from build123d import *

# Parameters (mm, degrees)
F0_R     = 48.25
F0_R_2   = 46.25
F0_R_3   = 43
F0_R_4   = 41
F1_DEPTH = 5
F2_DEPTH = 4.75
F3_SIZE  = 0.3


with BuildPart() as f1:
    # F0 (on Front) → F1 (new body, symmetric)
    with BuildSketch(Plane.XZ):
        Circle(F0_R)
        Circle(F0_R_2, mode=Mode.SUBTRACT)
        Circle(F0_R_3)
        Circle(F0_R_4, mode=Mode.SUBTRACT)
    extrude(amount=F1_DEPTH, both=True)

    # F0 (on Front) → F2 (join, symmetric)
    with BuildSketch(Plane.XZ):
        Circle(F0_R_2)
        Circle(F0_R_3, mode=Mode.SUBTRACT)
    extrude(amount=F2_DEPTH, both=True)

    # F3
    f3_edges = [f1.edges().sort_by_distance(p)[0] for p in [
        (-48.25, 5, 0),
        (48.25, 0, 0),
        (-48.25, -5, 0),
        (-41, -5, 0),
        (41, 0, 0),
        (-41, 5, 0),
    ]]
    chamfer(f3_edges, length=F3_SIZE)


solid = f1.part
CAD build for the part. Positions are in the model's coordinates, mm. A direction names the side the tool comes from. Round coordinates to 2 decimals unless told otherwise and drop trailing zeros. Loops run counter-clockwise (first coordinate to the right, second up) from the corner with the lowest first, then second, coordinate; pieces in that order, holes last. Notation, with made-up numbers: (-20, 88) - (29, 88) arc R15 ccw to (29, 97) - close; hole circle Ø1 at (2, 65.5). An arc over 180 degrees is marked (long way). Put each result on its own line as item: value.
1. Wall check: line 1 (Z direction, x = 0, y = 4.8); line 2 (Z direction, x = 0, y = -4.9); line 3 (Z direction, x = -0.5, y = 1.75). Give the ranges that are in metal, low to high.
Geometry check:
line 1: -48.15 to -46.25, -43 to -41.1, 41.1 to 43, 46.25 to 48.15
line 2: -48.05 to -46.25, -43 to -41.2, 41.2 to 43, 46.25 to 48.05
line 3: -48.25 to -41, 41 to 48.25
2. Slice it at C-C on y = 3.25. List the corners of the cut face in (x, z).
Geometry check:
outline: circle Ø96.5 at (0, 0); hole circle Ø82 at (0, 0)
3. Pin check, flat tips, straight feed: P1, Ø2, axis at y = 1.5, z = 17.5, coming from the +X side; P2, Ø4, axis at y = -1.5, z = -25.5, coming from the -X side; P3, Ø3, axis at x = -25, y = 3.5, coming from the +Z side. Stop position of each tip, or through.
Geometry check:
P1: x = 45.34
P2: x = -42.14
P3: z = 42.14
4. 3-axis set-ups, long thin cutter, end or side, ignore diameter. For faces 3 (the flat face through (-25.1, -5, 39.3)), 4 (the flat face through (31, 4.75, -31)), 5 (the flat face through (31, -4.75, -31)): which of +Z, -Z, +X, -X, +Y, -Y reach the whole face in a straight line?
Geometry check:
face 3: +Z, -Z, +X, -X, -Y
face 4: +Y
face 5: -Y
5. Two-plate mould, pull along Z, no slides. Class faces 1 (the flat face through (-25.1, 5, 39.3)), 2 (the cylindrical face through (-9, 0, -40)): released by +Z, released by -Z, zero draft, split by the parting line, or undercut.
Geometry check:
face 1: zero draft
face 2: undercut
